Autodesk Inventor part; units mm, degrees
ref_plane "Work Plane1" through (0, 7, 0) normal (0, 1, 0) x (1, 0, 0)
ref_plane "YZ Plane" through (0, 0, 0) normal (1, 0, 0) x (0, 1, 0)
ref_plane "XZ Plane" through (0, 0, 0) normal (0, 1, 0) x (-1, 0, 0)
sketch "Sketch1" plane through (0, 0, 0) normal (0, 1, 0) x (-1, 0, 0)
  arc A0 (-20.2731, 67) -> (-20.2731, -67) centre (0, 0) ccw
  line L0 (0, 67) -> (0, -67)
  line L1 (0, -67) -> (-20.2731, -67)
  line L2 (-20.2731, 67) -> (-20.2731, -67)
  line L3 (-20.2731, 0) -> (-0.2731, 0)
  circle A1 centre (-0.2731, 0) radius 20
  circle A2 centre (-0.2731, 0) radius 15
  line L4 (-20.2731, 20) -> (69.7269, 20)
  arc A3 (66.8089, -20) -> (66.8089, 20) centre (-0.2731, 0) ccw
  line L5 (-20.2731, -20) -> (66.8089, -20)
  dimension "d0" = 140
  dimension "d1" = 134
  dimension "d2" = 20
  dimension "d3" = 30
  dimension "d4" = 90
extrude "Extrusion1" add sketch "Sketch1" against normal blind 29 contours L2 A0 | L4 A1 L2 | L2 A1 L5 | A1 L0 A2 L3 | L3 A2 L0 A1 | A1 L0 A2 | L4 A3 L5 A1 | A2 L0 | A2 L0
sketch "Sketch2" plane through (0, 0, 0) normal (0, 1, 0) x (1, 0, 0)
  line L0 (-66.8089, 20) -> (20.2731, 20)
  line L1 (20.2731, -20.1759) -> (20.2731, 20)
  line L2 (20.2731, -20.1759) -> (-74.6075, -20.1759)
  line L3 (-74.6075, -20.1759) -> (-74.6075, 20)
  line L4 (-74.6075, 20) -> (20.2731, 20)
  line L5 (20.2731, 20) -> (20.2731, -20.1759)
  point P0 (0, 0)
extrude "Extrusion2" cut sketch "Sketch2" against normal blind 10
ref_plane "Work Plane1" through (0, 7, 0) normal (0, 1, 0) x (1, 0, 0)
sketch "Sketch3" plane through (0, -29, 0) normal (0, -1, 0) x (1, 0, 0)
  line L0 (20.2731, -67) -> (20.2731, 67)
  line L1 (20.2731, 0) -> (0.2731, 0)
  circle A0 centre (0.2731, 0) radius 20
  point P0 (0, 0)
  dimension "d10" = 20
extrude "Extrusion3" add sketch "Sketch3" along normal blind 30
sketch "Sketch4" plane through (0.2731, -59, 0) normal (0, -1, 0) x (1, 0, 0)
  point P0 (-0.2731, 0)
sketch "Sketch5" plane through (0, -29, 0) normal (0, -1, 0) x (1, 0, 0)
  line L0 (20.2731, -67) -> (20.2731, 67)
  line L1 (20.2731, 0) -> (0.2731, 0)
  circle A0 centre (0.2731, 0) radius 15
  point P0 (0, 0)
  dimension "d13" = 20
  dimension "d14" = 30
extrude "Extrusion4" add sketch "Sketch5" along normal blind 90
sketch "Sketch6" plane through (0, 0, 0) normal (0, 1, 0) x (1, 0, 0)
  point P0 (0, 0)
sketch "Sketch7" plane through (0, -10, 0) normal (0, 1, 0) x (1, 0, 0)
  line L0 (20.2731, 67) -> (20.2731, -67)
  line L1 (20.2731, 0) -> (-49.7269, 0)
  circle A0 centre (-49.7269, 0) radius 15
  point P0 (0, 0)
  dimension "d17" = 70
  dimension "d18" = 30
extrude "Extrusion5" add sketch "Sketch7" along normal blind 17
mirror "Mirror1" about plane through (0, 7, 0) normal (0, 1, 0) of "Extrusion1", "Extrusion5", "Extrusion3", "Extrusion4", "Extrusion2"
hole "Hole1" at (-49.7269, 43, 0) direction (0, -1, 0) diameter 14 end through all
sketch "Sketch8" plane through (0, 7, 0) normal (0, 1, 0) x (1, 0, 0)
  arc A0 (0.2731, -20) -> (0.2731, 20) centre (0.2731, 0) ccw
  line L0 (20.2731, 0) -> (0.2731, 0)
  circle A1 centre (0.2731, 0) radius 15
  point P0 (0, 0)
  dimension "d30" = 20
properties part number "crank"
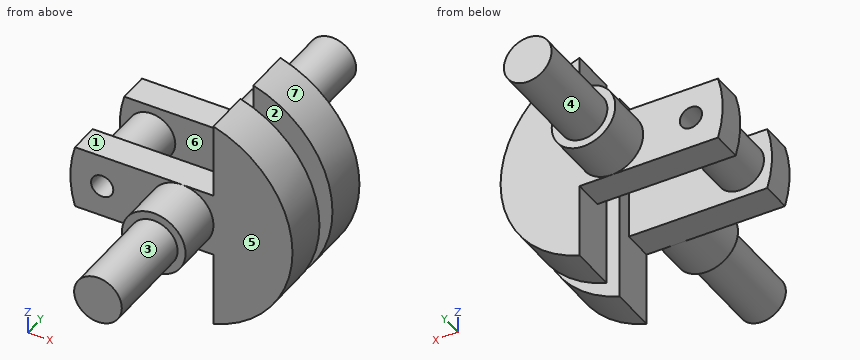
Here's how the part is built. I have some questions about the finished solid (model axes, mm). Face numbers are marked on the shaded views. A direction names the side the tool comes from. Give positions to 0.01 mm unless a question says otherwise; leave off trailing zeros. Order: outer loops, then holes, each group sorted by start corner. A loop starts at its lowest first (then second) coordinate and runs counter-clockwise, first axis right, second up. Notation, with made-up numbers: (-17, -18) -> (18, -18) arc R19 cw to (18, -9) -> close; hole circle Ø1 at (66.5, 0). An arc over 180 degrees is marked (long way). Use a Markdown table: item, result. Add a question column.
Item 1: Imagine slicing it at B-B on z = -46. Please give me the cut outline in (x, y), plus the area to 3 significant figures.
Item 2: Imagine slicing it at D-D on x = -11.5. Please give me the cut outline in (y, z), plus the area to 3 significant figures.
Item 3: Will these pins go through, and if not, where does the flat tip stop? pin 1 (8 mm diameter, centred on x = 44, z = 5, fed in from +Y); pin 2 (9.5 mm diameter, centred on x = -41.5, y = -22.5, fed in from -Z); pin 3 (20 mm diameter, centred on x = -50.5, z = 8, fed in from -Y).
Item 4: If we mould it in two halves opening along X, with no side actions, what happens to the marked faces 5, 6 and 7? For each: pulls with the +X half, pulls with the -X half, needs draft (parallel to the pull), parting line crosses it, or undercut.
Item 5: For the marked faces 1, 2, 3 and 4, which set-ups out of +Z, -Z, +X, -X, +Y, -Y let a thin tool reach every point of the face, with its end or its side?
Item 6: Imagine slicing it at C-C on y = 84.5. Please give me the cut outline in (x, z).
Item 7: I need wall thicknesses on line 1 (X direction, y = 1.5, z = 0); line 2 (Y direction, x = -8.5, z = -4); line 3 (Y direction, x = -43, z = 15). Which ranges of each line are inside material? Lowest first, please.
Item 8: Imagine slicing it at A-A on x = -26.5. Please give me the cut outline in (y, z), plus the area to 3 significant figures.
Data:
| question | item | result |
|---|---|---|
| 1 | outline | (20.27, -29) -> (52.76, -29) -> (52.76, 0) -> (20.27, 0) -> close; (20.27, 14) -> (52.76, 14) -> (52.76, 43) -> (20.27, 43) -> close |
| 1 | area | 1,880 mm² |
| 2 | outline | (-119, -9.29) -> (-59, -9.29) -> (-59, -16.17) -> (-29, -16.17) -> (-29, -20) -> (-10, -20) -> (-10, 20) -> (-29, 20) -> (-29, 16.17) -> (-59, 16.17) -> (-59, 9.29) -> (-119, 9.29) -> close; (24, -20) -> (43, -20) -> (43, -16.17) -> (73, -16.17) -> (73, -9.29) -> (133, -9.29) -> (133, 9.29) -> (73, 9.29) -> (73, 16.17) -> (43, 16.17) -> (43, 20) -> (24, 20) -> close |
| 2 | area | 5,690 mm² |
| 3 | pin 1 | stops at y = 43 |
| 3 | pin 2 | stops at z = -20 |
| 3 | pin 3 | stops at y = -29 |
| 4 | face 5 | needs draft |
| 4 | face 6 | undercut |
| 4 | face 7 | pulls with the +X half |
| 5 | face 1 | +Z, -X, +Y, -Y |
| 5 | face 2 | +Z, -Z, +X |
| 5 | face 3 | -Y |
| 5 | face 4 | +Y |
| 6 | outline | circle Ø30 at (0.27, 0) |
| 7 | line 1 | x = -64.73 to -56.73, -42.73 to -34.73 |
| 7 | line 2 | y = -119 to -10, 24 to 133 |
| 7 | line 3 | y = -29 to -10, 24 to 43 |
| 8 | outline | (-29, -20) -> (-10, -20) -> (-10, 20) -> (-29, 20) -> close; (24, -20) -> (43, -20) -> (43, 20) -> (24, 20) -> close |
| 8 | area | 1,520 mm² |
